```python
from build123d import *

# Parameters (mm, degrees)
SKETCH1_W           = 80
SKETCH1_H           = 200
BOSS_EXTRUDE1_DEPTH = 5
SKETCH2_W           = 20
SKETCH2_H           = 5
BOSS_EXTRUDE2_DEPTH = 5


with BuildPart() as part:
    # Sketch1 → Boss-Extrude1 (new body)
    with BuildSketch(Plane.XY):
        with Locations((-40, 100)):
            Rectangle(SKETCH1_W, SKETCH1_H)
    extrude(amount=BOSS_EXTRUDE1_DEPTH)

    # Sketch2 → Boss-Extrude2 (add)
    with BuildSketch(Plane.XY.offset(5)):
        with Locations((-20, 202.5)):
            Rectangle(SKETCH2_W, SKETCH2_H)
        with Locations((-60, 202.5)):
            Rectangle(SKETCH2_W, SKETCH2_H)
        with Locations((-60, -2.5)):
            Rectangle(SKETCH2_W, SKETCH2_H)
        with Locations((-20, -2.5)):
            Rectangle(SKETCH2_W, SKETCH2_H)
    extrude(amount=-BOSS_EXTRUDE2_DEPTH)


solid = part.part
```
Geometry: final body of the model. Coordinates: model frame, mm. A direction names the side the tool comes from. Coordinates: 2 decimals unless noted, no trailing zeros. Order: outer loops, then holes, each group sorted by start corner. A loop starts at its lowest first (then second) coordinate and runs counter-clockwise, first axis right, second up. Notation, with made-up numbers: (62.25, -5) -> (98.25, -5) arc R10 cw to (98.25, 1) -> close; hole circle Ø9 at (-2, -27). An arc over 180 degrees is marked (long way). Answer in a Markdown table with one row per item.
Item 1: Section A-A on z = 2.95. Output: boundary loops of the cut face in (x, y), plus the area to 3 significant figures.
Return value:
| item | result |
|---|---|
| outline | (-80, 0) -> (-70, 0) -> (-70, -5) -> (-50, -5) -> (-50, 0) -> (-30, 0) -> (-30, -5) -> (-10, -5) -> (-10, 0) -> (0, 0) -> (0, 200) -> (-10, 200) -> (-10, 205) -> (-30, 205) -> (-30, 200) -> (-50, 200) -> (-50, 205) -> (-70, 205) -> (-70, 200) -> (-80, 200) -> close |
| area | 16,400 mm² |
Item 2: Section B-B on x = -37. Output: boundary loops of the cut face in (y, z), plus the area to 3 significant figures.
Return value:
| item | result |
|---|---|
| outline | (0, 0) -> (200, 0) -> (200, 5) -> (0, 5) -> close |
| area | 1,000 mm² |
Item 3: Ray query, L1, parallel to Y at x = -32, z = 2.5. Return the intervals inside material, ascending.
Return value:
| item | result |
|---|---|
| L1 | y = 0 to 200 |
Item 4: Access query for faces 4 (the flat face through (-5, 200, 2)), 5 (the flat face through (-50, 202, 3)), 6 (the flat face through (-70, 202, 3)), 7 (the flat face through (-10, -3, 3)), 8 (the flat face through (-30, -3, 3)). Directions: +Z, -Z, +X, -X, +Y, -Y. A direction counts if a zero-diameter tool reaches every point of the face in a straight line with its end or side. Return the directions, or none.
Return value:
| item | result |
|---|---|
| face 4 | +Z, -Z, +X, +Y |
| face 5 | +Z, -Z, +Y |
| face 6 | +Z, -Z, -X, +Y |
| face 7 | +Z, -Z, +X, -Y |
| face 8 | +Z, -Z, -Y |
Item 5: Contact query for flat-ended pins moving along their axis: P1, Ø2.5, axis at x = -6.5, z = 1.5, coming from the +Y side; P2, Ø1, axis at x = -35, y = 90.5, coming from the -Z side; P3, Ø2.5, axis at x = -7.5, z = 2.5, coming from the -Y side. Output: stop coordinate, or through.
Return value:
| item | result |
|---|---|
| P1 | stops at y = 200 |
| P2 | stops at z = 0 |
| P3 | stops at y = 0 |
Item 6: Draft query along X for faces 1 (the flat face through (0, 99, 2)), 2 (the flat face through (-20, -5, 3)), 3 (the flat face through (-50, -3, 3)). Return one class per face: released by +X, released by -X, zero draft, split by the parting line, or undercut.
Return value:
| item | result |
|---|---|
| face 1 | released by +X |
| face 2 | zero draft |
| face 3 | undercut |
